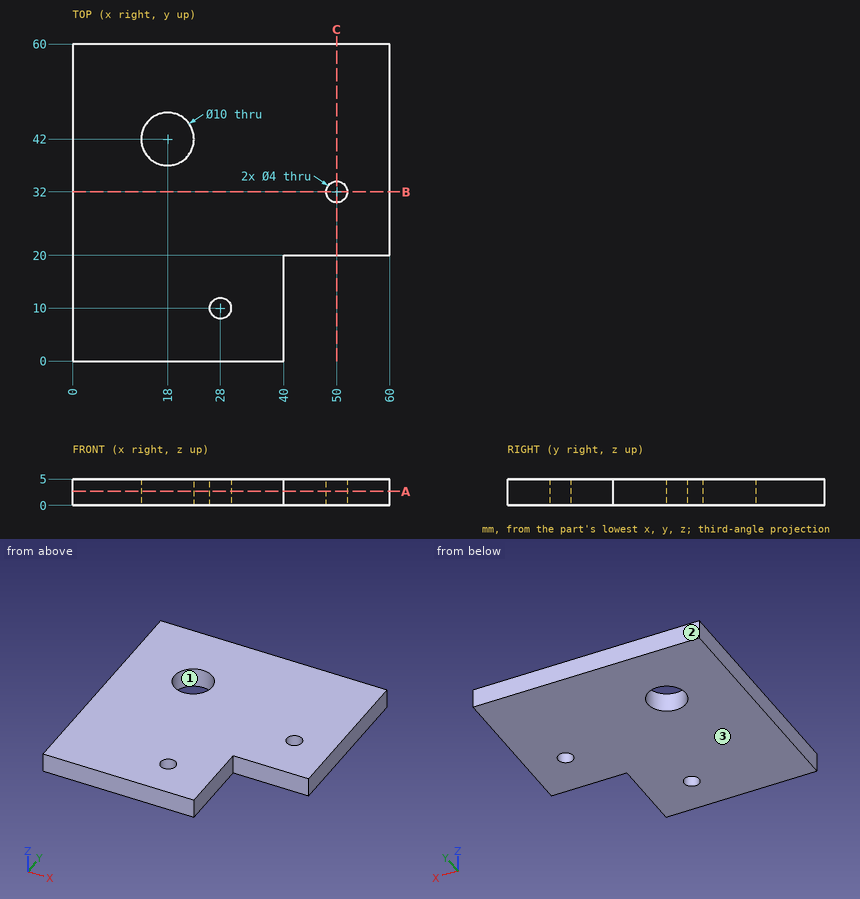
The drawing under review shows one solid part. Ordinate dimensions are in mm from its lowest x, y, z. Coordinates: 2 decimals unless noted, no trailing zeros. Write each loop counter-clockwise with the first axis right and the second up, starting at its lowest first coordinate (ties: lowest second). Pieces come first, ordered by that corner, then holes. Notation, with made-up numbers: M -19,30.5 L -13,30.5 A30 cw -13,69.5 Z; hole C -3.5,24.5 d6. An arc over 180 degrees is marked long. Answer as a JSON object with one key per item and string values.
Item 1: Wall thickness on probe 1 along Y at (x, z) = (50, 3.8); probe 2 along Y at (x, z) = (42.5, 0.3); probe 3 along X at (y, z) = (43, 4.1): over which ranges is each line inside the solid? List them lowest first.
Outcome:
{"probe 1": "20 to 30, 34 to 60", "probe 2": "20 to 60", "probe 3": "0 to 13.1, 22.9 to 60"}
Item 2: Add section C-C, the plane x = 50. Give the boundary of the cut face in (y, z).
Outcome:
{"outline": "M 20,0 L 30,0 L 30,5 L 20,5 Z; M 34,0 L 60,0 L 60,5 L 34,5 Z"}
Item 3: Add section A-A, the plane z = 2.65. Give the boundary of the cut face in (x, y).
Outcome:
{"outline": "M 0,0 L 40,0 L 40,20 L 60,20 L 60,60 L 0,60 Z; hole C 18,42 d10; hole C 28,10 d4; hole C 50,32 d4"}
Item 4: Draft analysis for pull direction Y (two halves, no side actions). For the marked faces 1, 2 and 3, state which applies: pulls with the +Y half, pulls with the -Y half, needs draft (parallel to the pull), parting line crosses it, or undercut.
Outcome:
{"face 1": "undercut", "face 2": "pulls with the +Y half", "face 3": "needs draft"}
Item 5: Insertion check: pin 1 Ø1.5 at (x, z) = (51.5, 2.5) entering from -Y. The pin has a flat end and moves straight along its axis. Give the tip position at first contact, or say it passes through.
Outcome:
{"pin 1": "y = 20"}
Item 6: Add section B-B, the plane y = 32. Give the boundary of the cut face in (x, z).
Outcome:
{"outline": "M 0,0 L 48,0 L 48,5 L 0,5 Z; M 52,0 L 60,0 L 60,5 L 52,5 Z"}
